Source: three-view drawing plus pictorial views. Frame: mm from the lowest corner of the part. A direction names the side the tool comes from. Round coordinates to 2 decimals unless told otherwise and drop trailing zeros. Loops run counter-clockwise (first coordinate to the right, second up) from the corner with the lowest first, then second, coordinate; pieces in that order, holes last. Notation, with made-up numbers: (62.5, 67.5) -> (73.5, 67.5) arc R15 cw to (73.5, 76.5) -> close; hole circle Ø2 at (-16.5, 69.25). An arc over 180 degrees is marked (long way). Answer in a Markdown table with one row per item.
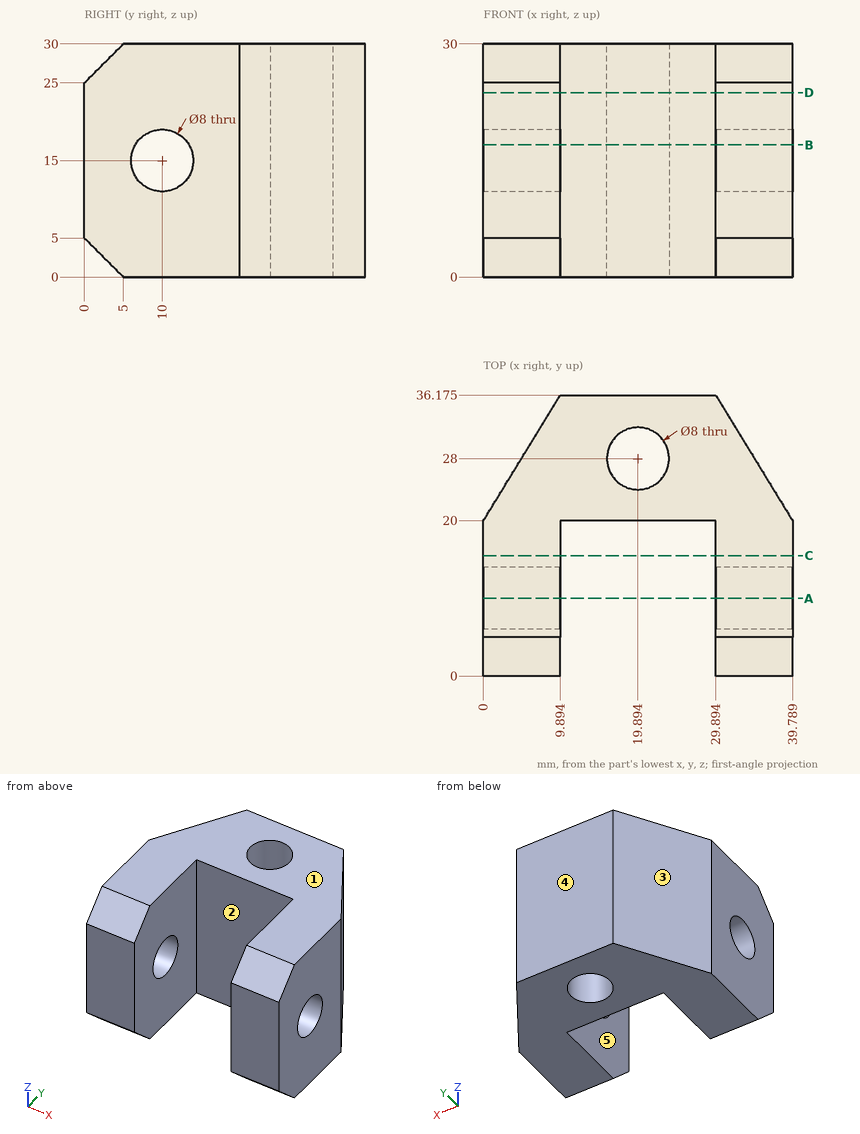
Item 1: Cut plane A-A (y = 10). Output: boundary loops of the cut face in (x, z) (1 decimal), then the cut area to 3 significant figures.
Answer:
| item | result |
|---|---|
| outline | (0, 0) -> (9.9, 0) -> (9.9, 11) -> (0, 11) -> close; (0, 19) -> (9.9, 19) -> (9.9, 30) -> (0, 30) -> close; (29.9, 0) -> (39.8, 0) -> (39.8, 11) -> (29.9, 11) -> close; (29.9, 19) -> (39.8, 19) -> (39.8, 30) -> (29.9, 30) -> close |
| area | 435 mm² |
Item 2: Line query: probe 1 along X at (y, z) = (18.5, 20.75) (1 decimal); probe 2 along Y at (x, z) = (18, 4.25) (1 decimal); probe 3 along Y at (x, z) = (11, 19) (1 decimal). Output: solid intervals per line, ascending. Write a range as [from, to].
Answer:
| item | result |
|---|---|
| probe 1 | x = [0, 9.9], [29.9, 39.8] |
| probe 2 | y = [20, 24.5], [31.5, 36.2] |
| probe 3 | y = [20, 36.2] |
Item 3: Cut plane D-D (z = 23.75). Output: boundary loops of the cut face in (x, y) (1 decimal), then the cut area to 3 significant figures.
Answer:
| item | result |
|---|---|
| outline | (0, 0) -> (9.9, 0) -> (9.9, 20) -> (29.9, 20) -> (29.9, 0) -> (39.8, 0) -> (39.8, 20) -> (29.9, 36.2) -> (9.9, 36.2) -> (0, 20) -> close; hole circle Ø8 at (19.9, 28) |
| area | 829 mm² |
Item 4: Reachability of the marked faces 1 and 2 from +Z, -Z, +X, -X, +Y, -Y: full face, straight path, thin tool, end or side. Return the list, or none.
Answer:
| item | result |
|---|---|
| face 1 | +Z, +X, -X, +Y, -Y |
| face 2 | +Z, -Z, -Y |
Item 5: Draft query along X for the marked faces 3, 4 and 5. Return one class per face: pulls with the +X half, pulls with the -X half, needs draft (parallel to the pull), parting line crosses it, or undercut.
Answer:
| item | result |
|---|---|
| face 3 | pulls with the -X half |
| face 4 | needs draft |
| face 5 | undercut |
Item 6: Cut plane B-B (z = 17). Output: boundary loops of the cut face in (x, y) (1 decimal), then the cut area to 3 significant figures.
Answer:
| item | result |
|---|---|
| outline | (0, 0) -> (9.9, 0) -> (9.9, 6.5) -> (0, 6.5) -> close; (0, 13.5) -> (9.9, 13.5) -> (9.9, 20) -> (29.9, 20) -> (29.9, 13.5) -> (39.8, 13.5) -> (39.8, 20) -> (29.9, 36.2) -> (9.9, 36.2) -> (0, 20) -> close; (29.9, 0) -> (39.8, 0) -> (39.8, 6.5) -> (29.9, 6.5) -> close; hole circle Ø8 at (19.9, 28) |
| area | 692 mm² |
Item 7: Pin query (flat end, axial travel): pin 1 Ø7 at (x, y) = (19.89, 28) entering from -Z; pin 2 Ø6 at (y, z) = (29, 23) entering from -X; pin 3 Ø3 at (y, z) = (25, 18) entering from -X; pin 4 Ø3 at (y, z) = (25.5, 4) entering from +X. Return the tip coordinate at first contact, or that it passes through.
Answer:
| item | result |
|---|---|
| pin 1 | passes through |
| pin 2 | stops at x = 3.67 |
| pin 3 | stops at x = 2.14 |
| pin 4 | stops at x = 37.34 |
Item 8: Cut plane C-C (y = 15.5). Output: boundary loops of the cut face in (x, z) (1 decimal), then the cut area to 3 significant figures.
Answer:
| item | result |
|---|---|
| outline | (0, 0) -> (9.9, 0) -> (9.9, 30) -> (0, 30) -> close; (29.9, 0) -> (39.8, 0) -> (39.8, 30) -> (29.9, 30) -> close |
| area | 594 mm² |
